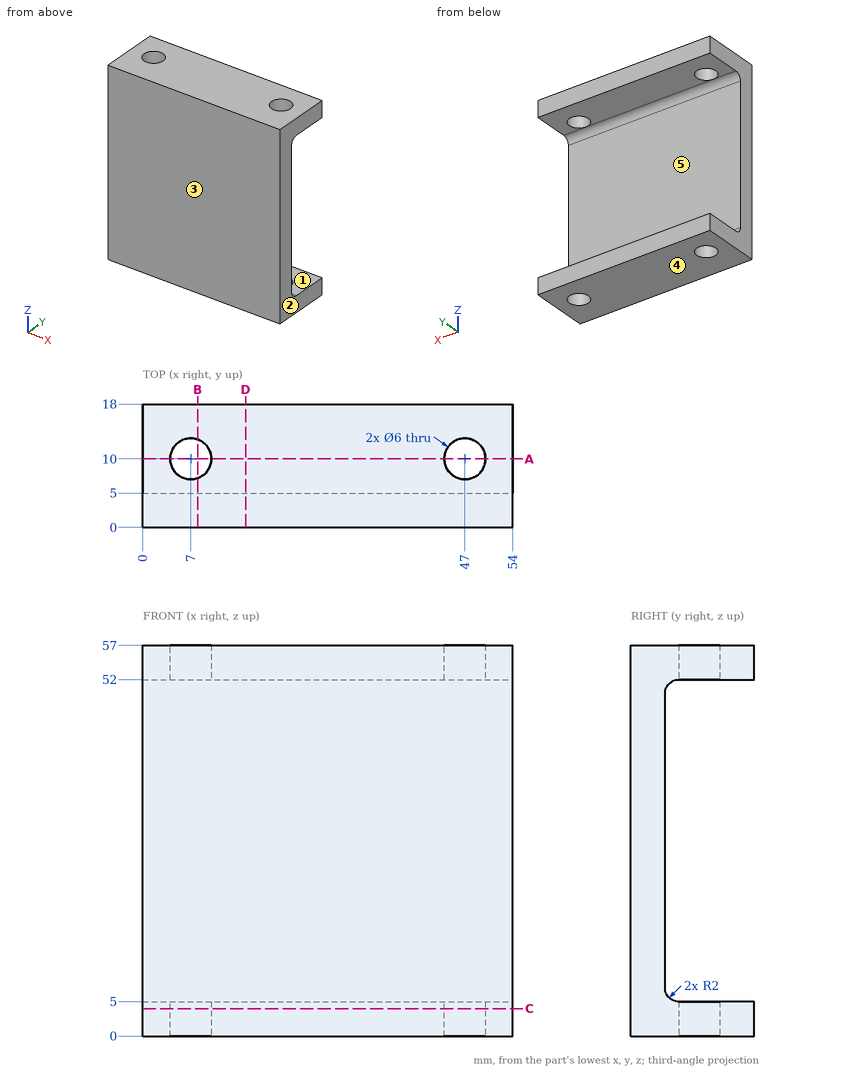
Job drawing, mm, ordinate dimensions from the low corner. One solid piece. A direction names the side the tool comes from. Round coordinates to 2 decimals unless told otherwise and drop trailing zeros. Loops run counter-clockwise (first coordinate to the right, second up) from the corner with the lowest first, then second, coordinate; pieces in that order, holes last.
Item 1: 3-axis set-ups, long thin cutter, end or side, ignore diameter. For the marked faces 1 and 2: which of +Z, -Z, +X, -X, +Y, -Y reach the whole face in a straight line?
Item 2: Cut at B-B, the plane x = 8. Give the cut face in (y, z), then the cut area to 3 significant figures.
Item 3: Cut at D-D, the plane x = 15. Give the cut face in (y, z), then the cut area to 3 significant figures.
Item 4: Cut at C-C, the plane z = 4. Give the cut face in (x, y).
Item 5: Cut at A-A, the plane y = 10. Give the cut face in (x, z).
Item 6: Drop flat-ended pins along their axis: P1, Ø1, axis at x = 43.5, z = 30.5, coming from the +Y side; P2, Ø1, axis at x = 32.5, y = 5.5, coming from the -Z side. Give the stop position or say it passes through.
Item 7: Drill centre lines: line 1 (X direction, y = 10, z = 53.25); line 2 (Z direction, x = 6, y = 16.25); line 3 (Y direction, x = 47, z = 55). Where is each one in solid material? Low to high.
Item 8: Mould opens along Z. For the marked faces 3, 4 and 5 say: +Z half, -Z half, draft (parallel to the pull), parting line (faces both ways), or undercut.
A:
1. face 1: +X, -X, +Y
1. face 2: +Z, -Z, +X, +Y, -Y
2. outline: (0, 0) - (7.17, 0) - (7.17, 5) - (7, 5) arc R2 cw to (5, 7) - (5, 50) arc R2 cw to (7, 52) - (7.17, 52) - (7.17, 57) - (0, 57) - close; (12.83, 0) - (18, 0) - (18, 5) - (12.83, 5) - close; (12.83, 52) - (18, 52) - (18, 57) - (12.83, 57) - close
2. area: 360 mm2
3. outline: (0, 0) - (18, 0) - (18, 5) - (7, 5) arc R2 cw to (5, 7) - (5, 50) arc R2 cw to (7, 52) - (18, 52) - (18, 57) - (0, 57) - close
3. area: 417 mm2
4. outline: (0, 0) - (54, 0) - (54, 18) - (0, 18) - close; hole circle Ø6 at (7, 10); hole circle Ø6 at (47, 10)
5. outline: (0, 0) - (4, 0) - (4, 5) - (0, 5) - close; (0, 52) - (4, 52) - (4, 57) - (0, 57) - close; (10, 0) - (44, 0) - (44, 5) - (10, 5) - close; (10, 52) - (44, 52) - (44, 57) - (10, 57) - close; (50, 0) - (54, 0) - (54, 5) - (50, 5) - close; (50, 52) - (54, 52) - (54, 57) - (50, 57) - close
6. P1: stops at y = 5
6. P2: stops at z = 0
7. line 1: x = 0 to 4, 10 to 44, 50 to 54
7. line 2: z = 0 to 5, 52 to 57
7. line 3: y = 0 to 7, 13 to 18
8. face 3: draft
8. face 4: -Z half
8. face 5: undercut
